The drawing under review shows one solid part. Ordinate dimensions are in mm from its lowest x, y, z. Give positions to 0.01 mm unless a question says otherwise; leave off trailing zeros. Write each loop counter-clockwise with the first axis right and the second up, starting at its lowest first coordinate (ties: lowest second). Pieces come first, ordered by that corner, then holes. Notation, with made-up numbers: (-2, 40.5) -> (4, 40.5) arc R15 cw to (4, 50.5) -> close; hole circle Ø11 at (17.25, -3.5). An arc over 180 degrees is marked (long way). Use CSV: the item, a comma, the result in double quotes.
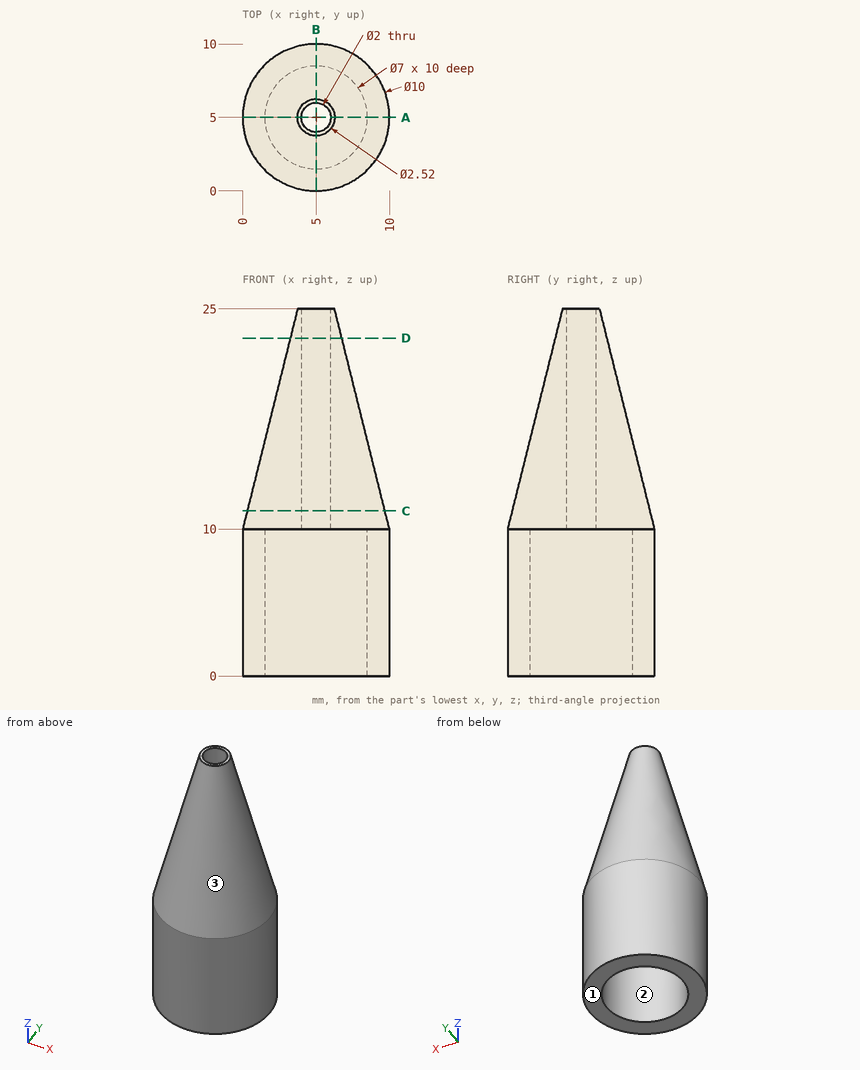
(1) For line 1 along Y through (x, z) = (5, 2.5); line 2 along Y through (x, z) = (8, 2.25); line 3 along X through (y, z) = (5, 14.25), list the stretches that pass through material, from the lowest coordinate up. Write a range as [from, to].
Established:
line 1,"y = [0, 1.5], [8.5, 10]"
line 2,"y = [1, 3.2], [6.8, 9]"
line 3,"x = [1.06, 4], [6, 8.94]"
(2) Clearance check with flat-ended pins moving along their axes: pin 1 (6 mm diameter, centred on x = 5, z = 22, fed in from -Y); pin 2 (2 mm diameter, centred on x = 5, z = 15.5, fed in from +Y); pin 3 (1 mm diameter, centred on y = 3, z = 19.5, fed in from -X). State where each tip first meets the part, or that it passes through.
Established:
pin 1,"stops at y = 2.24"
pin 2,"stops at y = 8.88"
pin 3,"stops at x = 2.81"
(3) Take a section at D-D (z = 23). Write out the cut boundary in (x, y).
Established:
outline,"circle Ø3.52 at (5, 5); hole circle Ø2 at (5, 5)"
(4) Take a section at C-C (z = 11.25). Write out the cut boundary in (x, y).
Established:
outline,"circle Ø9.38 at (5, 5); hole circle Ø2 at (5, 5)"
(5) Mouldability with a two-part tool opening along Y and no side actions: class the marked faces 1, 2 and 3 as +Y half, -Y half, draft (parallel to the pull), parting line (faces both ways), or undercut.
Established:
face 1,"draft"
face 2,"undercut"
face 3,"parting line"
(6) Take a section at A-A (y = 5). Write out the cut boundary in (x, z), then the cut area to 3 significant figures.
Established:
outline,"(0, 0) -> (1.5, 0) -> (1.5, 10) -> (4, 10) -> (4, 25) -> (3.74, 25) -> (0, 10) -> close; (6, 10) -> (8.5, 10) -> (8.5, 0) -> (10, 0) -> (10, 10) -> (6.26, 25) -> (6, 25) -> close"
area,"93.9 mm2"
